```python
from build123d import *

# Parameters (mm, degrees)
F1_DEPTH = 63.5
F2_DEPTH = 25.4
F3_DEPTH = 7.9375


with BuildPart() as f1:
    # F0 (on Front) → F1 (new body, symmetric)
    with BuildSketch(Plane.XZ):
        Polygon((-41.275, 9.525), (-41.275, -9.525), (41.275, -9.525), (41.275, 9.525), (22.225, 9.525), align=None)
    extrude(amount=F1_DEPTH, both=True)

    # F0 (on Front) → F2 (join, symmetric)
    with BuildSketch(Plane.XZ):
        with BuildLine():
            Line((22.225, 9.525), (41.275, 9.525))
            Line((41.275, 9.525), (41.275, 27.0002))
            ThreePointArc((41.275, 27.0002), (45.92468, 38.22552), (57.15, 42.8752))
            Line((57.15, 42.8752), (61.991871, 42.8752))
            Line((61.991871, 42.8752), (61.991871, 61.9252))
            Line((61.991871, 61.9252), (57.15, 61.9252))
            add(Edge.make_bspline(
                [(55.007715, 61.859435), (55.727449, 61.887292), (56.441689, 61.909225), (57.15, 61.9252)],
                knots=[109.507647, 109.507647, 109.507647, 109.507647, 111.504536, 111.504536, 111.504536, 111.504536], degree=3))
            ThreePointArc((55.007715, 61.859435), (31.708155, 50.926507), (22.225, 27.0002))
            Line((22.225, 27.0002), (22.225, 9.525))
        make_face()
    extrude(amount=F2_DEPTH, both=True)

    # F0 (on Front) → F3 (join, symmetric)
    with BuildSketch(Plane.XZ):
        with BuildLine():
            add(Edge.make_bspline(
                [(-41.275, 9.525), (-40.454127, 40.988729), (15.538124, 60.331766), (55.007715, 61.859435)],
                knots=[0, 0, 0, 0, 109.507647, 109.507647, 109.507647, 109.507647], degree=3))
            Line((-41.275, 9.525), (22.225, 9.525))
            Line((22.225, 9.525), (22.225, 27.0002))
            ThreePointArc((22.225, 27.0002), (31.708155, 50.926507), (55.007715, 61.859435))
        make_face()
    extrude(amount=F3_DEPTH, both=True)


solid = f1.part
```
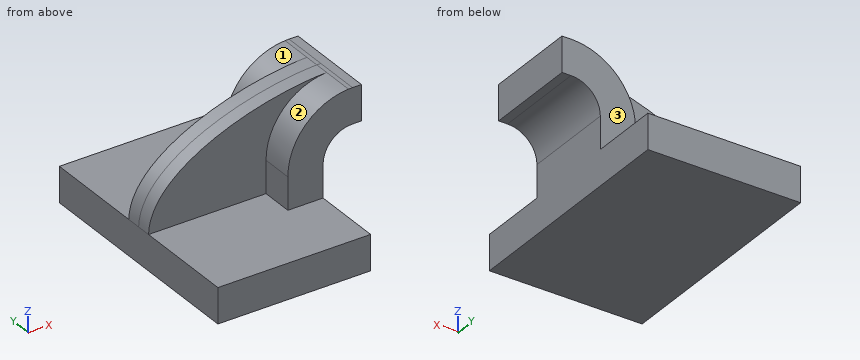
Source: CAD feature listing. Evaluate the final solid. Frame: model axes, mm. Face numbers are marked on the shaded views. A direction names the side the tool comes from. Give positions to 0.01 mm unless a question says otherwise; leave off trailing zeros. Write each loop counter-clockwise with the first axis right and the second up, starting at its lowest first coordinate (ties: lowest second). Pieces come first, ordered by that corner, then holes. Notation, with made-up numbers: (29, 66) - (39, 66) arc R7 cw to (39, 75) - close; hole circle Ø11 at (87, 2.5). An arc over 180 degrees is marked (long way). One line per item, written item: value. Start each with the question number.
Q1. Section query A-A, the plane z = 6.5. Return the cut outline in (x, y) (3 decimals), then the cut area to 3 significant figures.
Q2. First-contact query: pin 1 Ø1 at (x, y) = (6.5, -32) entering from +Z (3 decimals); pin 2 Ø19 at (y, z) = (18.5, 17) entering from -X (3 decimals); pin 3 Ø1.5 at (x, z) = (-24.5, 39.5) entering from -Y; pin 4 Ø1.5 at (x, y) = (16.5, -1.5) entering from +Z. Flat tips, straight axial feed; report the tip coordinate or a pass-through.
Q3. Section query B-B, the plane y = -30.5. Return the cut outline in (x, z) (3 decimals), then the cut area to 3 significant figures.
Q4. Set-up query: the marked faces 1, 2 and 3. Return all of +Z, -Z, +X, -X, +Y, -Y with unobstructed straight access to the full face (end or side cutting, diameter ignored); none if empty.
Q5. Material intervals for probe 1 along Y at (x, z) = (14.5, 27); probe 2 along Z at (x, y) = (9, -27.5) (3 decimals); probe 3 along X at (y, z) = (-21, 13) (3 decimals), sorted ascending. Write a range as from..to.
Answer:
1. outline: (-41.275, -63.5) - (41.275, -63.5) - (41.275, 63.5) - (-41.275, 63.5) - close
1. area: 10,500 mm2
2. pin 1: stops at z = 9.525
2. pin 2: stops at x = -41.275
2. pin 3: passes through
2. pin 4: stops at z = 55.91
3. outline: (-41.275, -9.525) - (41.275, -9.525) - (41.275, 9.525) - (-41.275, 9.525) - close
3. area: 1,570 mm2
4. face 1: +Z, -X, +Y
4. face 2: +Z, -X, -Y
4. face 3: +Z, +X, -X, +Y
5. probe 1: y = -7.94..7.94
5. probe 2: z = -9.525..9.525
5. probe 3: x = 22.225..41.275
